Solid Edge part; units mm, degrees
sketch "Sketch1" plane through (0, 0, 0) normal (0, -1, 0) x (1, 0, 0)
  line L0 (0, -6) -> (1.5, -6)
  line L1 (1.5, -6) -> (1.5, -0.601)
  line L2 (1.5, -0.601) -> (1.3375, -0.101)
  line L3 (1.3375, -0.101) -> (1.3375, 0)
  line L4 (1.3375, 0) -> (2.8, 0)
  line L5 (2.8, 0) -> (2.6425, 1.8)
  line L6 (2.6425, 1.8) -> (0, 1.8)
  dimension "D1" = 1.3375
  dimension "D2" = 1.5
  dimension "D3" = 2.6425
revolve "RevolvedProtrusion1" add sketch "Sketch1" angle 360 about axis through (0, 0, 6) along (0, 0, -1)
fillet "Round_1" radius 0.9 1 edges at (-2.6425, 0, 1.8)
sketch "Sketch2" plane through (0, 0, 0) normal (0, -1, 0) x (1, 0, 0)
  line L0 (-0.4, 1.8) -> (-0.4, 1.1)
  line L1 (-0.4, 1.1) -> (0.4, 1.1)
  line L2 (0.4, 1.1) -> (0.4, 1.8)
  line L3 (0.4, 1.8) -> (-0.4, 1.8)
  dimension "D1" = 0.4
  dimension "D2" = 0.4
extrude "ExtrudedCutout_1" cut sketch "Sketch2" along normal mid plane 5.6
cosmetic_thread "Thread_1" thread depth 5.399
fillet "Round_2" radius 0.1 1 edges at (-1.3375, 0, 0)
chamfer "Chamfer_1" distance 0.0012 angle 30 1 edges at (-1.5, 0, -6) measured on face at (1.03, 0.97, -6)
properties material "Steel"
The listing builds one solid part. Answer for the finished solid, in the listing's coordinates (mm). A direction names the side the tool comes from. Coordinates: 2 decimals unless noted, no trailing zeros. Write each loop counter-clockwise with the first axis right and the second up, starting at its lowest first coordinate (ties: lowest second). Pieces come first, ordered by that corner, then holes. Notation, with made-up numbers: (15.5, -14) - (67.5, -14) arc R18 ccw to (67.5, 16) - close; hole circle Ø11 at (66.25, 15.25). An arc over 180 degrees is marked (long way). Return JSON: item names as keys, results as strings. Group by question number.
Q1. Flat-ended cylindrical pins translate along their axes: pin 1 Ø2 at (x, z) = (1.5, -2.5) entering from +Y; pin 2 Ø3 at (x, z) = (-1.5, -0.5) entering from +Y; pin 3 Ø1.5 at (x, z) = (2, -1.5) entering from -Y. Find the tip coordinate at first contact, or state that the pin passes through.
Q2. The part is cut by section C-C on z = -4.5. Write down the section's boundary in (x, y), and give its area (3 significant figures).
Q3. For a pull along X with two mould halves and no side action, classify faces 1 (the conical face through (-2.17, 1.67, 0.7)), 2 (the flat face through (-1, 0, 1.8)), 3 (the flat face through (0, 0, 1.1)) as +X half, -X half, draft (parallel to the pull), parting line (faces both ways), or undercut.
Q4. Which of the six approach directions +Z, -Z, +X, -X, +Y, -Y give full straight-line access (tool end or side, diameter ignored) to faces 4 (the cylindrical face through (-1.5, 0.07, -3.26)), 5 (the flat face through (1, 0, 1.8))?
Q5. Find the intervals of material crossed by line 1 along Z through (x, y) = (-0.25, -1.2); line 2 along Y through (x, z) = (0.1, -1.75), in increasing order. Write a range as [from, to].
Evaluation:
{
 "1": {"pin 1": "stops at y = 1.41", "pin 2": "stops at y = 2.8", "pin 3": "stops at y = -0.83"},
 "2": {"outline": "circle Ø3 at (0, 0)", "area": "7.07 mm2"},
 "3": {"face 1": "parting line", "face 2": "draft", "face 3": "undercut"},
 "4": {"face 4": "-Z", "face 5": "+Z, +X, -X, +Y, -Y"},
 "5": {"line 1": "z = [-6, 1.1]", "line 2": "y = [-1.5, 1.5]"}
}
